Verification items for the finished model (mm, model axes). A direction names the side the tool comes from. Round coordinates to 2 decimals unless told otherwise and drop trailing zeros. Order: outer loops, then holes, each group sorted by start corner. A loop starts at its lowest first (then second) coordinate and runs counter-clockwise, first axis right, second up.
```python
from build123d import *

# Parameters (mm, degrees)
SKETCH040_W    = 27
SKETCH040_H    = 23
PAD011_DEPTH   = 6
SKETCH041_R    = 8
HOLE013_DEPTH  = 25
SKETCH042_R    = 1.1
HOLE014_DEPTH  = 25
SKETCH043_R    = 0.8
HOLE015_DEPTH  = 3.519312
HOLE015_TIPS_R = 0.8


with BuildPart() as fix:
    # Sketch040 → Pad011 (new body)
    with BuildSketch(Plane.XZ):
        with Locations((-42.54, 19.462705)):
            Rectangle(SKETCH040_W, SKETCH040_H)
    extrude(amount=PAD011_DEPTH)

    # Sketch041 (on Face6 of Pad011) → Hole013 (cut)
    with BuildSketch(Plane.XZ.offset(6)):
        with Locations((-42.54, 20.462705)):
            Circle(SKETCH041_R)
    extrude(amount=-HOLE013_DEPTH, mode=Mode.SUBTRACT)

    # Sketch042 (on Face5 of Hole013) → Hole014 (cut)
    with BuildSketch(Plane.XZ.offset(6)):
        with Locations((-50.54, 28.462705)):
            Circle(SKETCH042_R)
        with Locations((-34.54, 28.462705)):
            Circle(SKETCH042_R)
        with Locations((-50.54, 12.462705)):
            Circle(SKETCH042_R)
        with Locations((-34.54, 12.462705)):
            Circle(SKETCH042_R)
    extrude(amount=-HOLE014_DEPTH, mode=Mode.SUBTRACT)

    # Sketch043 (on Face6 of Hole014) → Hole015 (cut)
    with BuildSketch(Plane(origin=(0, 0, 7.962705), x_dir=(1, 0, 0), z_dir=(0, 0, -1))):
        with Locations((-53.04, 3)):
            Circle(SKETCH043_R)
        with Locations((-46.04, 3)):
            Circle(SKETCH043_R)
        with Locations((-39.04, 3)):
            Circle(SKETCH043_R)
        with Locations((-32.04, 3)):
            Circle(SKETCH043_R)
    extrude(amount=-HOLE015_DEPTH, mode=Mode.SUBTRACT)

    # Hole015 tips → Hole015 tip 1 section 0
    with BuildSketch(Plane(origin=(0, 0, 11.482016), x_dir=(1, 0, 0), z_dir=(0, 0, -1)), mode=Mode.PRIVATE) as hole015_tip_1_s0:
        with Locations((-53.04, 3)):
            Circle(HOLE015_TIPS_R)
    loft([hole015_tip_1_s0.sketch, Vertex(-53.04, -3, 11.962705)], mode=Mode.SUBTRACT)

    # Hole015 tips → Hole015 tip 2 section 0
    with BuildSketch(Plane(origin=(0, 0, 11.482016), x_dir=(1, 0, 0), z_dir=(0, 0, -1)), mode=Mode.PRIVATE) as hole015_tip_2_s0:
        with Locations((-46.04, 3)):
            Circle(HOLE015_TIPS_R)
    loft([hole015_tip_2_s0.sketch, Vertex(-46.04, -3, 11.962705)], mode=Mode.SUBTRACT)

    # Hole015 tips → Hole015 tip 3 section 0
    with BuildSketch(Plane(origin=(0, 0, 11.482016), x_dir=(1, 0, 0), z_dir=(0, 0, -1)), mode=Mode.PRIVATE) as hole015_tip_3_s0:
        with Locations((-39.04, 3)):
            Circle(HOLE015_TIPS_R)
    loft([hole015_tip_3_s0.sketch, Vertex(-39.04, -3, 11.962705)], mode=Mode.SUBTRACT)

    # Hole015 tips → Hole015 tip 4 section 0
    with BuildSketch(Plane(origin=(0, 0, 11.482016), x_dir=(1, 0, 0), z_dir=(0, 0, -1)), mode=Mode.PRIVATE) as hole015_tip_4_s0:
        with Locations((-32.04, 3)):
            Circle(HOLE015_TIPS_R)
    loft([hole015_tip_4_s0.sketch, Vertex(-32.04, -3, 11.962705)], mode=Mode.SUBTRACT)


with BuildPart() as fix_1:
    # Body006021004 placement: moved
    add(fix.part.moved(Location((0, -105.83, -1.96))))


with BuildPart() as part_mirroring001:
    # Part__Mirroring001: instance of Fix
    add(fix_1.part.mirror(Plane(origin=(0, 0, 0), x_dir=(0, -1, 0), z_dir=(1, 0, 0))))


with BuildPart() as part_mirroring001_1:
    # Part__Mirroring001 placement: moved
    add(part_mirroring001.part.moved(Location((-56, 0, 16))))


solid = part_mirroring001_1.part
```
1) Go/stop test with flat-tipped pins: pin 1 Ø1.8 at (x, y) = (-10, -108.5) entering from -Z; pin 2 Ø1 at (x, y) = (-2.96, -108.83) entering from -Z; pin 3 Ø4 at (x, z) = (-17.5, 35.5) entering from -Y; pin 4 Ø1.3 at (x, y) = (-9.96, -108.83) entering from -Z. Record where each tip stops, or that it passes through.
2) Sectioned sample at B-B on z = 35.5. Record the cut outline in (x, y), then the cut area to 3 significant figures.
3) Scan lines: probe 1 along X at (y, z) = (-108.83, 24.35); probe 2 along Z at (x, y) = (-13.46, -110.35); probe 3 along Z at (x, y) = (-4.5, -107.5). Record each from-to range of solid material in increasing order.
4) Tool access check on faces 5 (the cylindrical face through (-16.79, -108.05, 23.74)), 6 (the cylindrical face through (-5.317, -108.872, 43.593)). Record the directions out of +Z, -Z, +X, -X, +Y, -Y that give a thin tool (end or side, any length) a straight path to the whole face; none if there is none.
5) Draft check along Y on faces 1 (the cylindrical face through (-10.33, -108.12, 23.74)), 2 (the flat face through (-13, -105.83, 26)), 3 (the flat face through (0.04, -109, 33)), 4 (the flat face through (-13, -111.83, 26)). Enter one of: released by +Y, released by -Y, zero draft, split by the parting line, or undercut.
6) Sectioned sample at A-A on x = -13.46. Record the cut outline in (y, z).
7) Sectioned sample at C-C on y = -106.9. Record the cut outline in (x, z).
Returned:
1. pin 1: stops at z = 22
1. pin 2: stops at z = 25.7
1. pin 3: passes through
1. pin 4: stops at z = 25.61
2. outline: (-26.96, -111.83) - (-21.4, -111.83) - (-21.4, -105.83) - (-26.96, -105.83) - close; (-5.52, -111.83) - (0.04, -111.83) - (0.04, -105.83) - (-5.52, -105.83) - close
2. area: 66.7 mm2
3. probe 1: x = -26.96 to -24.76, -23.16 to -17.76, -16.16 to -10.76, -9.16 to -3.76, -2.16 to 0.04
3. probe 2: z = 22 to 26.5, 42.5 to 45
3. probe 3: z = 22 to 25.97, 27.04 to 41.97, 43.04 to 45
4. face 5: -Z
4. face 6: +Y, -Y
5. face 1: undercut
5. face 2: released by +Y
5. face 3: zero draft
5. face 4: released by -Y
6. outline: (-111.83, 22) - (-105.83, 22) - (-105.83, 26.5) - (-111.83, 26.5) - close; (-111.83, 42.5) - (-105.83, 42.5) - (-105.83, 45) - (-111.83, 45) - close
7. outline: (-26.96, 22) - (0.04, 22) - (0.04, 45) - (-26.96, 45) - close; hole circle Ø2.2 at (-21.46, 26.5); hole circle Ø2.2 at (-21.46, 42.5); hole circle Ø16 at (-13.46, 34.5); hole circle Ø2.2 at (-5.46, 26.5); hole circle Ø2.2 at (-5.46, 42.5)
